```python
from build123d import *
from OCP.BRepFilletAPI import BRepFilletAPI_MakeChamfer

# Parameters (mm, degrees)
SKETCH1_R                = 0.85
BOSS_EXTRUDE1_DEPTH      = 5
BOSS_EXTRUDE2_DEPTH      = 2
SKETCH3_R                = 2.25
BOSS_EXTRUDE3_DEPTH      = 5
SKETCH4_R                = 3.5
CUT_EXTRUDE1_DEPTH       = 3
SKETCH5_W                = 10
SKETCH5_H                = 10
CUT_EXTRUDE2_DEPTH       = 47.770717335
FILLET1_R                = 7
BOSS_EXTRUDE4_DEPTH      = 5
BOSS_EXTRUDE4_DEPTH_BACK = 8
SKETCH6_W                = 7.5
SKETCH6_H                = 25
SKETCH7_W                = 7
SKETCH7_H                = 14
BOSS_EXTRUDE5_DEPTH      = 27.5
SKETCH8_W                = 18.5
SKETCH8_H                = 14
BOSS_EXTRUDE6_DEPTH      = 6
CHAMFER3_SIZE            = 0.5
CHAMFER1_SIZE            = 2.5
CHAMFER1_SIZE_2          = 1.25


with BuildPart() as part:
    # Sketch1 → Boss-Extrude1 (new body)
    with BuildSketch(Plane.XY):
        Polygon((-10, -35), (-10, 30), (10, 30), (10, -35), (17.5, -35), (17.5, 37.5), (-17.5, 37.5), (-17.5, -35), align=None)
        with Locations((-12.5, 32.5)):
            Circle(SKETCH1_R, mode=Mode.SUBTRACT)
        with Locations((12.5, 32.5)):
            Circle(SKETCH1_R, mode=Mode.SUBTRACT)
    extrude(amount=BOSS_EXTRUDE1_DEPTH)

    # Sketch2 → Boss-Extrude2 (add)
    with BuildSketch(Plane.XY):
        Polygon((17.5, -35), (17.5, 37.5), (-17.5, 37.5), (-17.5, -35), (-15.1, -35), (-15.1, 35.1), (15.1, 35.1), (15.1, -35), align=None)
    extrude(amount=-BOSS_EXTRUDE2_DEPTH)

    # Sketch3 → Boss-Extrude3 (add)
    # profile 1 of 2: a face of its own
    with BuildSketch(Plane.XY):
        with BuildLine():
            Line((22.5, 5), (17.5, 5))
            Line((17.5, 5), (17.5, -5))
            Line((17.5, -5), (22.5, -5))
            ThreePointArc((22.5, -5), (27.5, 0), (22.5, 5))
        make_face()
        with Locations(Location((22.5, 0, 0), (0, 0, 180))):
            Circle(SKETCH3_R, mode=Mode.SUBTRACT)
    # profile 2 of 2: a face of its own
    with BuildSketch(Plane.XY):
        with BuildLine():
            Line((-22.5, 5), (-17.5, 5))
            Line((-17.5, 5), (-17.5, -5))
            Line((-17.5, -5), (-22.5, -5))
            ThreePointArc((-22.5, -5), (-27.5, 0), (-22.5, 5))
        make_face()
        with Locations(Location((-22.5, 0, 0), (0, 0, 180))):
            Circle(SKETCH3_R, mode=Mode.SUBTRACT)
    extrude(amount=BOSS_EXTRUDE3_DEPTH)

    # Sketch4 → Cut-Extrude1 (cut)
    with BuildSketch(Plane(origin=(0, 0, 0), x_dir=(-1, 0, 0), z_dir=(0, 0, -1))):
        with Locations((-22.5, 0)):
            Circle(SKETCH4_R)
        with Locations((22.5, 0)):
            Circle(SKETCH4_R)
    extrude(amount=-CUT_EXTRUDE1_DEPTH, mode=Mode.SUBTRACT)

    # Sketch5 → Cut-Extrude2 (cut, through all)
    with BuildSketch(Plane(origin=(0, 0, 0), x_dir=(-1, 0, 0), z_dir=(0, 0, -1))):
        with Locations((-12.5, 32.5)):
            Rectangle(SKETCH5_W, SKETCH5_H)
        with Locations((12.5, 32.5)):
            Rectangle(SKETCH5_W, SKETCH5_H)
    extrude(amount=CUT_EXTRUDE2_DEPTH, mode=Mode.SUBTRACT)

    # Fillet1
    fillet1_edges = [part.edges().sort_by_distance(p)[0] for p in [
        (-17.5, 37.5, 2.5),
        (17.5, 37.5, 2.5),
    ]]
    fillet(fillet1_edges, radius=FILLET1_R)

    # Sketch6 → Boss-Extrude4 (add, two sides: drawn at the far end of the back side and taken through both)
    with BuildSketch(Plane.XY.offset(-BOSS_EXTRUDE4_DEPTH_BACK)):
        with Locations((-13.75, -47.5)):
            Rectangle(SKETCH6_W, SKETCH6_H)
    extrude(amount=BOSS_EXTRUDE4_DEPTH + BOSS_EXTRUDE4_DEPTH_BACK)

    # Sketch7 → Boss-Extrude5 (add)
    with BuildSketch(Plane(origin=(-10, 0, 0), x_dir=(0, 0, -1), z_dir=(1, 0, 0))):
        with Locations((-1.5, -53)):
            Rectangle(SKETCH7_W, SKETCH7_H)
    extrude(amount=BOSS_EXTRUDE5_DEPTH)

    # Sketch8 → Boss-Extrude6 (add)
    with BuildSketch(Plane(origin=(0, 0, -2), x_dir=(-1, 0, 0), z_dir=(0, 0, -1))):
        with Locations((-8.25, -53)):
            Rectangle(SKETCH8_W, SKETCH8_H)
    extrude(amount=BOSS_EXTRUDE6_DEPTH)

    # Chamfer3
    chamfer3_edges = [part.edges().sort_by_distance(p)[0] for p in [
        (0, 30, 5),
        (-17.5, -32.5, 5),
        (0, 37.5, 5),
        (15.449747468, 35.449747468, 5),
        (-15.449747468, 35.449747468, 5),
        (0, -60, 5),
        (10, -2.5, 5),
        (-10, -8, 5),
        (17.5, -53, 5),
        (3.75, -46, 5),
        (13.75, -35, 5),
        (-13.35, 32.5, 0),
        (-13.35, 32.5, 5),
        (17.5, -20, 5),
        (11.65, 32.5, 0),
        (11.65, 32.5, 5),
        (27.5, 0, 5),
        (20, 5, 5),
        (20, -5, 5),
        (24.75, 0, 5),
        (-27.5, 0, 5),
        (-20, -5, 5),
        (-20, 5, 5),
        (-20.25, 0, 5),
    ]]
    chamfer(chamfer3_edges, length=CHAMFER3_SIZE)

    # Chamfer1
    chamfer1_edges_1 = [part.edges().sort_by_distance(p)[0] for p in [
        (26, 0, 3),
    ]]
    chamfer1_side_1 = [part.faces().sort_by_distance(p)[0] for p in [
        (26, 0, 2.975),
    ]]
    chamfer1_edges_2 = [part.edges().sort_by_distance(p)[0] for p in [
        (-19, 0, 3),
    ]]
    chamfer1_side_2 = [part.faces().sort_by_distance(p)[0] for p in [
        (-19, 0, 2.975),
    ]]
    chamfer1 = BRepFilletAPI_MakeChamfer(part.part.solid().wrapped)
    for e in chamfer1_edges_1:
        chamfer1.Add(CHAMFER1_SIZE - 0.0001, CHAMFER1_SIZE_2 - 0.0001, e.wrapped, chamfer1_side_1[0].wrapped)
    for e in chamfer1_edges_2:
        chamfer1.Add(CHAMFER1_SIZE - 0.0001, CHAMFER1_SIZE_2 - 0.0001, e.wrapped, chamfer1_side_2[0].wrapped)
    add(Compound.cast(chamfer1.Shape()), mode=Mode.REPLACE)  # a hair under: the kernel refuses the full size


solid = part.part
```
Work out the finished part from the listing and answer in its coordinate system (mm). A direction names the side the tool comes from. Give positions to 0.01 mm unless a question says otherwise; leave off trailing zeros. Order: outer loops, then holes, each group sorted by start corner. A loop starts at its lowest first (then second) coordinate and runs counter-clockwise, first axis right, second up. Notation, with made-up numbers: M 72,20.25 L 84,20.25 A29 cw 84,58.25 Z; hole C 19,40.5 d10. An arc over 180 degrees is marked long. Return JSON: item names as keys, results as strings.
1) Section C-C, the plane z = -5.5 is taken. Write down the section's boundary in (x, y).
Resolved:
{"outline": "M -17.5,-60 L -10,-60 L -10,-35 L -17.5,-35 Z; M -1,-60 L 17.5,-60 L 17.5,-46 L -1,-46 Z"}
2) Section D-D, the plane y = -48.5 is taken. Write down the section's boundary in (x, z).
Resolved:
{"outline": "M -17.5,-8 L -10,-8 L -10,-2 L -1,-2 L -1,-8 L 17.5,-8 L 17.5,4.5 L 17,5 L -17,5 L -17.5,4.5 Z"}
3) Straight lines are drawn through the part: line 1 along X through (y, z) = (-10, 3.5); line 2 along X through (y, z) = (32.5, 3.4); line 3 along Y through (x, z) = (22.5, 3.95). For each, find the intervals that lie inside material, in ascending order. Write a range as [from, to].
Resolved:
{"line 1": "[-17.5, -10], [10, 17.5]", "line 2": "[-17.21, -13.35], [-11.65, 11.65], [13.35, 17.21]", "line 3": "[-5, -2.25], [2.25, 5]"}
4) Each of these flat-tipped pins is pushed along its axis until it touches: pin 1 (6 mm diameter, centred on y = -41, z = -6, fed in from -X); pin 2 (2 mm diameter, centred on x = -12, z = -5, fed in from +Y); pin 3 (1.9 mm diameter, centred on x = -16.5, y = -10, fed in from -Z); pin 4 (12 mm diameter, centred on x = 21, y = 27, fed in from +Z). Where does it stop, or does it pass through?
Resolved:
{"pin 1": "x = -17.5", "pin 2": "y = -35", "pin 3": "z = -2", "pin 4": "z = 5"}
5) For a pull along Y with two mould halves and no side action, classify faces 4 (the flat face through (14, -35, 2)), 5 (the flat face through (-20, 5, 2)), 6 (the flat face through (10, -2, 2)), 7 (the flat face through (12, -15, 5)) as +Y half, -Y half, draft (parallel to the pull), parting line (faces both ways), or undercut.
Resolved:
{"face 4": "undercut", "face 5": "+Y half", "face 6": "undercut", "face 7": "draft"}
6) Section A-A, the plane x = 8.5 is taken. Write down the section's boundary in (y, z).
Resolved:
{"outline": "M -60,-8 L -46,-8 L -46,4.5 L -46.5,5 L -59.5,5 L -60,4.5 Z; M 30,0 L 37.5,0 L 37.5,4.5 L 37,5 L 30.5,5 L 30,4.5 Z"}
7) A tool of negligible diameter and unlimited length cuts with its end or side. For faces 1 (the flat face through (-15.1, -4, -1)), 2 (the flat face through (-7.5, 36, -1)), 3 (the flat face through (0, 36, -2)), from which of +Z, -Z, +X, -X, +Y, -Y can it reach the whole face along a straight path? Write none if from no direction.
Resolved:
{"face 1": "-Z, +Y", "face 2": "-Z, -X, +Y", "face 3": "-Z, +X, -X, +Y"}
8) Section B-B, the plane y = -26.5 is taken. Write down the section's boundary in (x, z), plus the area to 3 significant figures.
Resolved:
{"outline": "M -17.5,-2 L -15.1,-2 L -15.1,0 L -10,0 L -10,4.5 L -10.5,5 L -17,5 L -17.5,4.5 Z; M 10,0 L 15.1,0 L 15.1,-2 L 17.5,-2 L 17.5,4.5 L 17,5 L 10.5,5 L 10,4.5 Z", "area": "84.1 mm^2"}
